Input: part model. Units: mm. Frame: model coordinates. Round coordinates to 2 decimals unless told otherwise and drop trailing zeros. Loops run counter-clockwise (first coordinate to the right, second up) from the corner with the lowest first, then second, coordinate; pieces in that order, holes last.
(1) Line query: line 1 (X direction, y = 3.15, z = -5); line 2 (Z direction, x = 6, y = 1.45); line 3 (Z direction, x = 8, y = 0.5). Output: solid intervals per line, ascending.
(2) Cut plane B-B, the plane x = 5. Output: boundary loops of the cut face in (y, z), and give its area (3 significant figures).
(3) First-contact query: pin 1 Ø1.6 at (y, z) = (2.5, 0) entering from -X; pin 2 Ø1 at (y, z) = (3.5, -14.5) entering from +X; pin 3 Ø1 at (x, y) = (11, 1) entering from -Z. Flat tips, straight axial feed; report the tip coordinate or a pass-through.
(4) Cut plane C-C, the plane z = -34. Output: boundary loops of the cut face in (x, y), and give its area (3 significant figures).
(5) Cut plane A-A, the plane y = 1.05. Output: boundary loops of the cut face in (x, z).
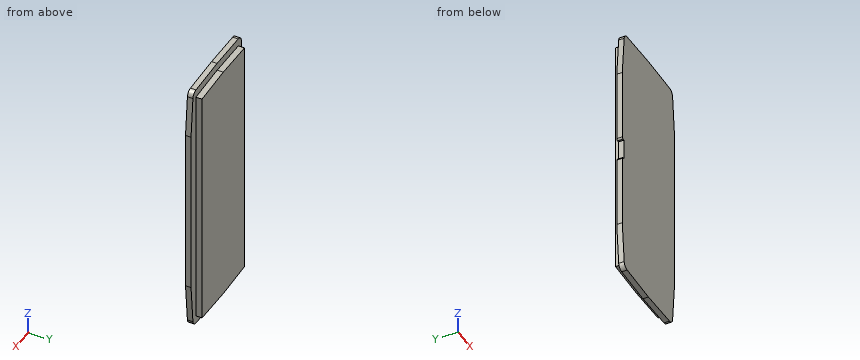
from build123d import *

# Parameters (mm, degrees)
EXTRUDE_1_DEPTH = 1.8
EXTRUDE_2_DEPTH = 3.8
FILLET_1_R      = 2


with BuildPart() as part:
    # Эскиз1 → Бобышка-Вытянуть1 (new body)
    with BuildSketch(Plane(origin=(0, 0, 0), x_dir=(1, 0, 0), z_dir=(0, 1, 0))):
        with BuildLine():
            Line((-15, 43.349382745), (-16.35, 28))
            Line((-16.35, 28), (-16.35, 4))
            ThreePointArc((-16.35, 4), (-16.203553391, 3.646446609), (-15.85, 3.5))
            Line((-15.85, 3.5), (-15.35, 3.5))
            Line((-15.35, 3.5), (-15.35, -3.5))
            Line((-15.35, -3.5), (-15.85, -3.5))
            ThreePointArc((-15.85, -3.5), (-16.203553391, -3.646446609), (-16.35, -4))
            Line((-16.35, -4), (-16.35, -28))
            Line((-16.35, -28), (-15, -43.35061617))
            Line((-15, -43.35061617), (0, -43.784698928))
            Line((0, -43.784698928), (15, -43.35061617))
            Line((15, -43.35061617), (16.35, -28))
            Line((16.35, -28), (16.35, 28))
            Line((16.35, 28), (15, 43.349382745))
            Line((15, 43.349382745), (0, 43.915301072))
            Line((0, 43.915301072), (-15, 43.349382745))
        make_face()
    extrude(amount=EXTRUDE_1_DEPTH)

    # Эскиз4 → Бобышка-Вытянуть2 (add)
    with BuildSketch(Plane(origin=(0, 0, 0), x_dir=(1, 0, 0), z_dir=(0, 1, 0))):
        Polygon((-13.3, 40.75), (-13.3, -40.75), (0, -41.25), (13.3, -40.75), (13.3, 40.75), (0, 41.25), align=None)
    extrude(amount=EXTRUDE_2_DEPTH)

    # Скругление1
    fillet_1_edges = [part.edges().sort_by_distance(p)[0] for p in [
        (-15, 0.9, -43.349382745),
        (15, 0.9, -43.349382745),
        (15, 0.9, 43.35061617),
        (-15, 0.9, 43.35061617),
    ]]
    fillet(fillet_1_edges, radius=FILLET_1_R)


solid = part.part
Reported:
1. line 1: x = -13.3 to 13.3
1. line 2: z = -43.69 to 43.61
1. line 3: z = -43.61 to 43.55
2. outline: (0, -43.73) - (1.8, -43.73) - (1.8, -41.06) - (3.8, -41.06) - (3.8, 41.06) - (1.8, 41.06) - (1.8, 43.64) - (0, 43.64) - close
2. area: 322 mm2
3. pin 1: stops at x = -15.35
3. pin 2: stops at x = 13.3
3. pin 3: stops at z = -43.52
4. outline: (-15.82, 0) - (15.82, 0) - (15.82, 1.8) - (13.3, 1.8) - (13.3, 3.8) - (-13.3, 3.8) - (-13.3, 1.8) - (-15.82, 1.8) - close
4. area: 110 mm2
5. outline: (-16.35, -28) - (-15.15, -41.59) arc R2 ccw to (-13.24, -43.42) - (0, -43.92) - (13.24, -43.42) arc R2 ccw to (15.15, -41.59) - (16.35, -28) - (16.35, 28) - (15.16, 41.58) arc R2 ccw to (13.22, 43.4) - (0, 43.78) - (-13.22, 43.4) arc R2 ccw to (-15.16, 41.58) - (-16.35, 28) - (-16.35, 4) arc R0.5 ccw to (-15.85, 3.5) - (-15.35, 3.5) - (-15.35, -3.5) - (-15.85, -3.5) arc R0.5 ccw to (-16.35, -4) - close
